Here's how the part is built. I have some questions about the finished solid (model axes, mm). Round coordinates to 2 decimals unless told otherwise and drop trailing zeros. Loops run counter-clockwise (first coordinate to the right, second up) from the corner with the lowest first, then second, coordinate; pieces in that order, holes last. Notation, with made-up numbers: M 41,-5.5 L 55,-5.5 A12 cw 55,4.5 Z; hole C 23.25,-25 d3. An arc over 180 degrees is marked long. Use a Markdown table: item, result.
Autodesk Inventor part; units mm, degrees
ref_plane "YZ Plane" through (0, 0, 0) normal (1, 0, 0) x (0, 1, 0)
ref_plane "XZ Plane" through (0, 0, 0) normal (0, 1, 0) x (-1, 0, 0)
ref_plane "XY Plane" through (0, 0, 0) normal (0, 0, 1) x (1, 0, 0)
sketch "Sketch1" plane through (0, 0, 0) normal (0, 0, 1) x (1, 0, 0)
  line L0 (-35, -6.5) -> (35, -6.5)
  line L1 (35, -6.5) -> (35, 6.5)
  line L2 (35, 6.5) -> (-35, 6.5)
  line L3 (-35, 6.5) -> (-35, -6.5)
  line L4 (-35, -6.5) -> (35, 6.5) construction
  line L5 (35, -6.5) -> (-35, 6.5) construction
  circle A0 centre (0, -16.5) radius 18
  line L6 (0, 6.5) -> (0, -6.5) construction
  point P0 (0, 0)
  point P1 (0, 0)
  point P2 (-14.9666, -6.5)
  point P3 (14.9666, -6.5)
  dimension "d0" = 36
  dimension "d1" = 10
  dimension "d2" = 70
  dimension "d3" = 13
extrude "Extrusion1" add sketch "Sketch1" along normal mid plane 60 contours L3 L2 L1 L0 A0
sketch "Sketch2" plane through (14.9666, -6.5, -30) normal (0, -1, 0) x (1, 0, 0)
  line L0 (-29.9333, 0) -> (-49.9666, 0)
  line L1 (-29.9333, 0) -> (-29.9333, 60)
  line L2 (-49.9666, 60) -> (-29.9333, 60)
  line L3 (-49.9666, 60) -> (-49.9666, 0)
  line L4 (20.0334, 0) -> (0, 0)
  line L5 (20.0334, 0) -> (20.0334, 60)
  line L6 (0, 60) -> (20.0334, 60)
  line L7 (0, 0) -> (0, 60)
  line L8 (-49.9666, 60) -> (-29.9333, 60)
  line L9 (-39.9499, 60) -> (-39.9499, 0)
  line L10 (-29.9333, 0) -> (-49.9666, 0)
  line L11 (20.0334, 0) -> (0, 0)
  line L12 (10.0167, 0) -> (10.0167, 60)
  line L13 (-49.9666, 30) -> (20.0334, 30) construction
  line L14 (-49.9666, 17.5) -> (20.0334, 17.5)
  line L15 (20.0334, 17.5) -> (20.0334, 42.5)
  line L16 (20.0334, 42.5) -> (-49.9666, 42.5)
  line L17 (-49.9666, 42.5) -> (-49.9666, 17.5)
  line L18 (-49.9666, 17.5) -> (20.0334, 42.5) construction
  line L19 (20.0334, 17.5) -> (-49.9666, 42.5) construction
  point P0 (-14.9666, 30)
  point P1 (-39.9499, 42.5)
  point P2 (-39.9499, 17.5)
  point P3 (10.0167, 17.5)
  point P4 (10.0167, 42.5)
  dimension "d6" = 25
hole "Hole1" at (-24.9833, -6.5, 12.5) at (-24.9833, -6.5, -12.5) at (24.9833, -6.5, -12.5) at (24.9833, -6.5, 12.5) direction (0, 1, 0) diameter 3.2 end through all
properties part number "19_Kep_han_B" material "ABS Plastic"
Q1. Imagine slicing it at B-B, the plane y = -2.5. Please give me the cut outline in (x, z), then the cut area to 3 significant figures.
Return value:
| item | result |
|---|---|
| outline | M -35,-30 L -11.31,-30 L -11.31,30 L -35,30 Z; M 11.31,-30 L 35,-30 L 35,30 L 11.31,30 Z; hole C -24.98,-12.5 d3.2; hole C -24.98,12.5 d3.2; hole C 24.98,-12.5 d3.2; hole C 24.98,12.5 d3.2 |
| area | 2,810 mm^2 |
Q2. I need wall thicknesses on line 1 (X direction, y = 2.25, z = 12.5); line 2 (Z direction, x = 24, y = 3); line 3 (X direction, y = -5.25, z = 12.5). Which ranges of each line are inside material? Lowest first, please. Write a range as from..to.
Return value:
| item | result |
|---|---|
| line 1 | x = -35..-26.58, -23.38..23.38, 26.58..35 |
| line 2 | z = -30..-13.76, -11.24..11.24, 13.76..30 |
| line 3 | x = -35..-26.58, -23.38..-14.05, 14.05..23.38, 26.58..35 |
Q3. Imagine slicing it at C-C, the plane z = 5.5. Please give me the cut outline in (x, y).
Return value:
| item | result |
|---|---|
| outline | M -35,-6.5 L -14.97,-6.5 A18 cw 14.97,-6.5 L 35,-6.5 L 35,6.5 L -35,6.5 Z |
Q4. Imagine slicing it at D-D, the plane x = -6. Please give me the cut outline in (y, z), then the cut area to 3 significant figures.
Return value:
| item | result |
|---|---|
| outline | M 0.47,-30 L 6.5,-30 L 6.5,30 L 0.47,30 Z |
| area | 362 mm^2 |
Q5. Imagine slicing it at A-A, the plane z = -12.5. Please give me the cut outline in (x, y).
Return value:
| item | result |
|---|---|
| outline | M -35,-6.5 L -26.58,-6.5 L -26.58,6.5 L -35,6.5 Z; M -23.38,-6.5 L -14.97,-6.5 A18 cw 14.97,-6.5 L 23.38,-6.5 L 23.38,6.5 L -23.38,6.5 Z; M 26.58,-6.5 L 35,-6.5 L 35,6.5 L 26.58,6.5 Z |
Q6. Will these pins go through, and if not, where does the flat tip stop? P1, Ø3.5, axis at x = -24.98, z = 12.5, coming from the +Y side; P2, Ø12, axis at x = 1.5, z = -23, coming from the -Y side; P3, Ø1.9, axis at x = 24.98, z = -12.5, coming from the -Y side.
Return value:
| item | result |
|---|---|
| P1 | stops at y = 6.5 |
| P2 | stops at y = -0.14 |
| P3 | passes through |
Q7. We'd pull the mould along X, two halves only. Please class faces 1 (the flat face through (-25, -6.5, 0)), 2 (the cylindrical face through (23.9, 0.09, -11.32)), 3 (the flat face through (-35, 0, 0)): pulls with the +X half, pulls with the -X half, needs draft (parallel to the pull), parting line crosses it, or undercut.
Return value:
| item | result |
|---|---|
| face 1 | needs draft |
| face 2 | undercut |
| face 3 | pulls with the -X half |
